Source: CAD feature listing. Evaluate the final solid. Frame: model axes, mm. A direction names the side the tool comes from. Give positions to 0.01 mm unless a question says otherwise; leave off trailing zeros. Answer in a Markdown table with one row per item.
```python
from build123d import *

# Parameters (mm, degrees)
F1_DEPTH = 20
F2_F1_R  = 9
F2_F2_R  = 9
F2_F3_R  = 9
F2_F4_R  = 9
F4_DEPTH = 50


# Not quite as in the source:
# - a feature names something its author has since deleted; it is built from what else it names


with BuildPart() as f1:
    # F0 (on Front) → F1 (new body)
    with BuildSketch(Plane.XZ):
        with BuildLine():
            ThreePointArc((2.6565660371, 12.138023602), (4.6349491554, 3.7302406753), (12.4253354109, 0))
            Line((12.4253354109, 0), (137.5746645891, 0))
            ThreePointArc((137.5746645891, 0), (145.3650508446, 3.7302406753), (147.3434339629, 12.138023602))
            Line((147.3434339629, 12.138023602), (135, 68.5359789614))
            ThreePointArc((135, 68.5359789614), (75, 100), (15, 68.5359789614))
            Line((15, 68.5359789614), (2.6565660371, 12.138023602))
        make_face()
    extrude(amount=F1_DEPTH)

    # F2: fillet of radius 9 on 13 edges, made by hand

    # F2_f1
    f2_f1_edges = [f1.edges().sort_by_distance(p)[0] for p in [
        (135, -10, 68.5359789614),
    ]]
    fillet(f2_f1_edges, radius=F2_F1_R)

    # F2_f2
    f2_f2_edges = [f1.edges().sort_by_distance(p)[0] for p in [
        (15, -10, 68.5359789614),
    ]]
    fillet(f2_f2_edges, radius=F2_F2_R)

    # F2_f3
    f2_f3_edges = [f1.edges().sort_by_distance(p)[0] for p in [
        (75, 0, 100),
    ]]
    fillet(f2_f3_edges, radius=F2_F3_R)

    # F2_f4
    f2_f4_edges = [f1.edges().sort_by_distance(p)[0] for p in [
        (75, -20, 100),
    ]]
    fillet(f2_f4_edges, radius=F2_F4_R)

    # F3 (on face) → F4 (cut)
    with BuildSketch(Plane(origin=(0, 0, 0), x_dir=(1, 0, 0), z_dir=(0, 0, -1))):
        with BuildLine():
            Line((29.25, 5.75), (120.75, 5.75))
            ThreePointArc((120.75, 5.75), (125, 10), (120.75, 14.25))
            Line((120.75, 14.25), (29.25, 14.25))
            ThreePointArc((29.25, 14.25), (25, 10), (29.25, 5.75))
        make_face()
    extrude(amount=-F4_DEPTH, mode=Mode.SUBTRACT)


solid = f1.part
```
(1) Access query for faces 4 (the flat face through (74, -10, 50)), 5 (the flat face through (74, -20, 41)). Directions: +Z, -Z, +X, -X, +Y, -Y. A direction counts if a zero-diameter tool reaches every point of the face in a straight line with its end or side. Return the directions, or none.
A:
| item | result |
|---|---|
| face 4 | -Z |
| face 5 | +Z, -Z, +X, -X, -Y |
(2) First-contact query: pin 1 Ø2 at (y, z) = (-4.5, 84.5) entering from +X; pin 2 Ø4 at (x, y) = (78, -11) entering from -Z; pin 3 Ø3 at (x, y) = (50.5, -4) entering from -Z. Flat tips, straight axial feed; report the tip coordinate or a pass-through.
A:
| item | result |
|---|---|
| pin 1 | stops at x = 119.54 |
| pin 2 | stops at z = 50 |
| pin 3 | stops at z = 0.71 |
(3) Pull-direction query (X, two-part tool) for faces 1 (the flat face through (74, 0, 41)), 2 (the flat face through (141.45, -9.99, 39.06)), 3 (the flat face through (76, -14.25, 25)); classes: +X half, -X half, draft (parallel to the pull), parting line (faces both ways), or undercut.
A:
| item | result |
|---|---|
| face 1 | draft |
| face 2 | +X half |
| face 3 | undercut |
(4) Ray query, probe 1 along Y at (x, z) = (113, 31); probe 2 along X at (y, z) = (-12.25, 49); probe 3 along X at (y, z) = (-10.5, 44). Return the intervals inside material, ascending.
A:
| item | result |
|---|---|
| probe 1 | y = -20 to -14.25, -5.75 to 0 |
| probe 2 | x = 10.81 to 25.64, 124.36 to 139.19 |
| probe 3 | x = 9.63 to 25.03, 124.97 to 140.37 |
